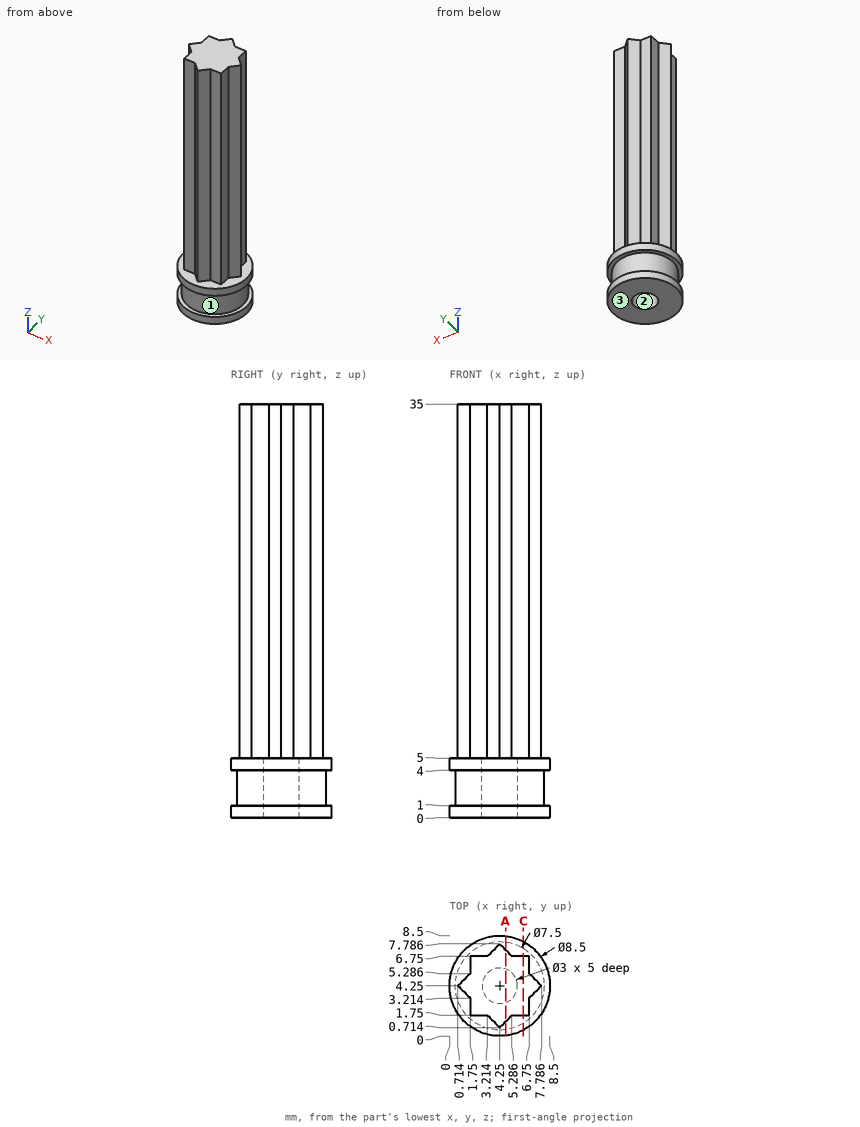
Study the drawing (mm; zero at the part's minimum x, y, z) and answer. Give positions to 0.01 mm unless a question says otherwise; leave off trailing zeros. Write each loop counter-clockwise with the first axis right and the second up, starting at its lowest first coordinate (ties: lowest second). Pieces come first, ordered by that corner, then holes. Notation, with made-up numbers: (-18, 88.25) -> (10, 88.25) arc R28 cw to (10, 119.25) -> close; hole circle Ø9 at (-30.75, 15.5). An arc over 180 degrees is marked (long way). Answer as a JSON object with one key per item and string values. Group by question number.
1) The mould has two halves that part along X. Classify the marked faces 1, 2 and 3: +X half, -X half, draft (parallel to the pull), parting line (faces both ways), or undercut.
2) Find section C-C (x = 6.25). Write down the section's boundary in (y, z), and give its area (3 significant figures).
3) Consider L1, parallel to Z at x = 7.5, y = 1.75; L2, parallel to Y at x = 4.25, z = 3.2; L3, parallel to X at y = 2, z = 8. Determine where each line is inside the solid, lowest interval first. Write a range as from..to.
4) Find section A-A (x = 4.75). Write down the section's boundary in (y, z) (1 decimal), and give its area (3 significant figures).
5) Each of these flat-tipped pins is pushed along its axis until it touches: P1, Ø0.7, axis at x = 2.5, z = 15.5, coming from the +Y side; P2, Ø0.9, axis at x = 4, y = 4.5, coming from the -Z side; P3, Ø2.5, axis at x = 5, y = 3, coming from the -Z side; P4, Ø0.7, axis at x = 6, z = 13.5, coming from the -Y side. Where does it stop, or does it pass through?
Values follow:
{
 "1": {"face 1": "parting line", "face 2": "undercut", "face 3": "draft"},
 "2": {"outline": "(0.5, 0) -> (8, 0) -> (8, 1) -> (7.42, 1) -> (7.42, 4) -> (8, 4) -> (8, 5) -> (6.75, 5) -> (6.75, 35) -> (1.75, 35) -> (1.75, 5) -> (0.5, 5) -> (0.5, 4) -> (1.08, 4) -> (1.08, 1) -> (0.5, 1) -> close", "area": "184 mm2"},
 "3": {"L1": "z = 0..1, 4..5", "L2": "y = 0.5..2.75, 5.75..8", "L3": "x = 1.75..6.75"},
 "4": {"outline": "(0, 0) -> (2.8, 0) -> (2.8, 5) -> (5.7, 5) -> (5.7, 0) -> (8.5, 0) -> (8.5, 1) -> (8, 1) -> (8, 4) -> (8.5, 4) -> (8.5, 5) -> (7.3, 5) -> (7.3, 35) -> (1.2, 35) -> (1.2, 5) -> (0, 5) -> (0, 4) -> (0.5, 4) -> (0.5, 1) -> (0, 1) -> close", "area": "207 mm2"},
 "5": {"P1": "stops at y = 6.75", "P2": "stops at z = 5", "P3": "stops at z = 0", "P4": "stops at y = 1.75"}
}
